Input: dimensioned drawing with shaded views. Units: mm. Origin: part minimum x, y, z. Round coordinates to 2 decimals unless told otherwise and drop trailing zeros. Loops run counter-clockwise (first coordinate to the right, second up) from the corner with the lowest first, then second, coordinate; pieces in that order, holes last. Notation, with made-up numbers: M 33.5,70 L 62.5,70 A9 ccw 62.5,83 Z; hole C 61,-18 d5. An arc over 180 degrees is marked long. Write each question's results on one line, items separated by ' | '. Start each with the question number.
1. Section A-A on z = 6. Output: boundary loops of the cut face in (x, y).
2. Section D-D on z = 9. Output: boundary loops of the cut face in (x, y), and give its area (3 significant figures).
3. Ray query, line 1 (X direction, y = 5.25, z = 6); line 2 (Y direction, x = 8, z = 11.5). Return the intervals inside material, ascending.
4. Draft query along X for the marked faces 1, 2 and 3. Return one class per face: released by +X, released by -X, zero draft, split by the parting line, or undercut.
5. Section B-B on x = 6. Output: boundary loops of the cut face in (y, z).
6. Contact query for flat-ended pins moving along their axis: pin 1 Ø1 at (y, z) = (6.5, 2) entering from -X; pin 2 Ø1 at (x, z) = (5.5, 4.5) entering from -Y; pin 3 Ø1 at (x, y) = (4, 3.5) entering from -Z; pin 4 Ø1.5 at (y, z) = (6, 2) entering from +X. Output: stop coordinate, or through.
7. Section C-C on y = 1.5. Output: boundary loops of the cut face in (x, z), and give its area (3 significant figures).
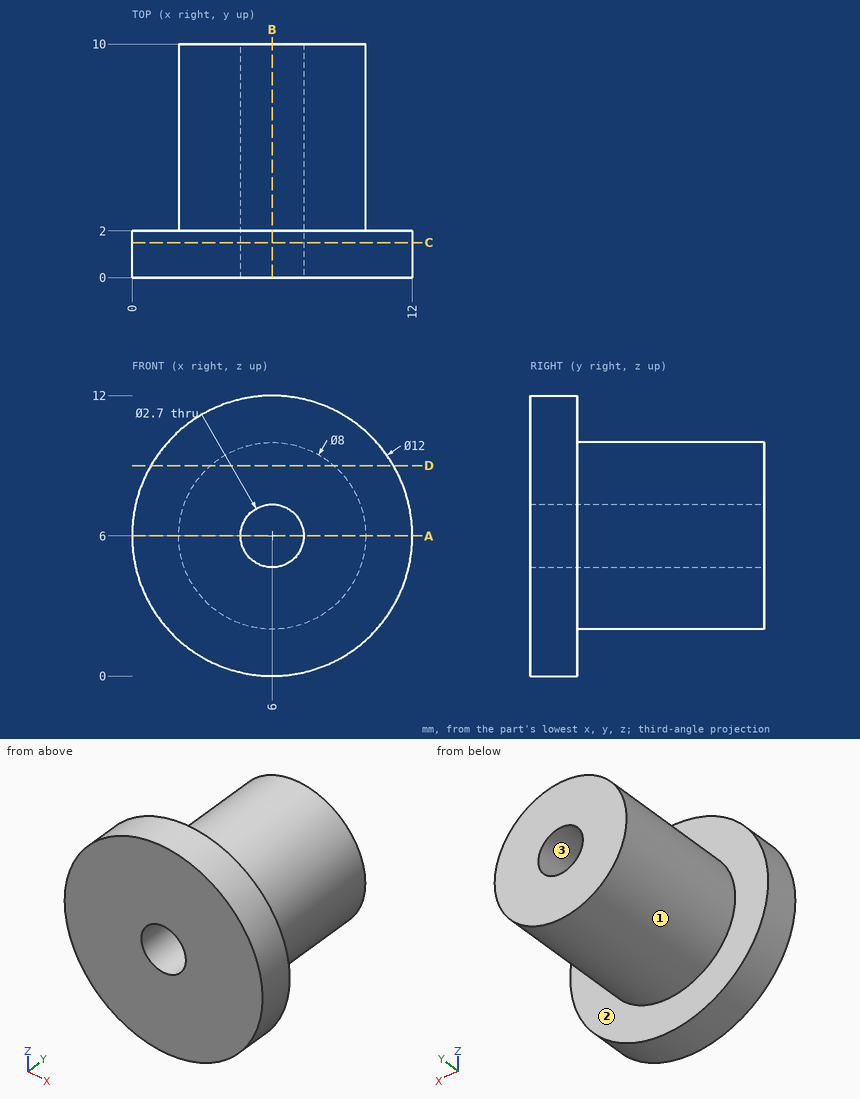
Taken from the geometry:
1) outline: M 0,0 L 4.65,0 L 4.65,10 L 2,10 L 2,2 L 0,2 Z; M 7.35,0 L 12,0 L 12,2 L 10,2 L 10,10 L 7.35,10 Z
2) outline: M 0.8,0 L 11.2,0 L 11.2,2 L 8.65,2 L 8.65,10 L 3.35,10 L 3.35,2 L 0.8,2 Z | area: 63.1 mm^2
3) line 1: 2 to 4.65, 7.35 to 10 | line 2: 0 to 2
4) face 1: split by the parting line | face 2: zero draft | face 3: undercut
5) outline: M 0,0 L 2,0 L 2,2 L 10,2 L 10,4.65 L 0,4.65 Z; M 0,7.35 L 10,7.35 L 10,10 L 2,10 L 2,12 L 0,12 Z
6) pin 1: x = 4.06 | pin 2: y = 0 | pin 3: z = 2.29 | pin 4: x = 8.33
7) outline: C 6,6 d12; hole C 6,6 d2.7 | area: 107 mm^2
